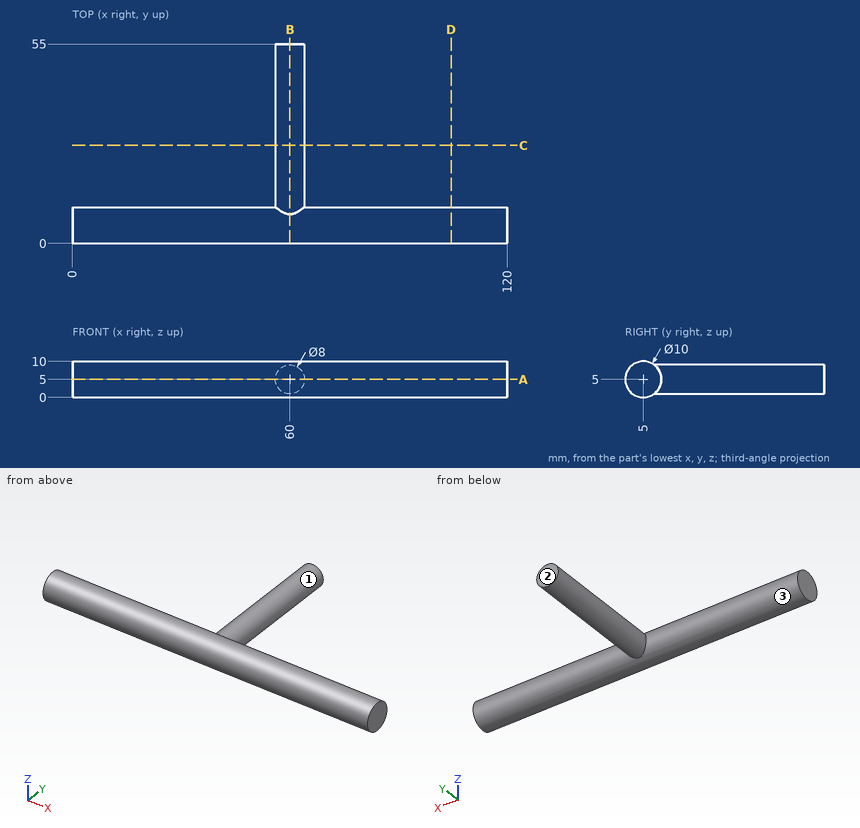
For this review, use the dimensioned drawing (mm, ordinates from the lowest corner) and the shaded views. A direction names the side the tool comes from. Give positions to 0.01 mm unless a question says otherwise; leave off trailing zeros. Write each loop counter-clockwise with the first axis right and the second up, starting at its lowest first coordinate (ties: lowest second). Pieces come first, ordered by that corner, then holes. Notation, with made-up numbers: M 82,-29 L 109,-29 A18 cw 109,-1 Z; hole C 43,54 d6. An arc over 180 degrees is marked long. Answer as a JSON object with one key per item and string values. Group by question number.
1) Clearance check with flat-ended pins moving along their axes: pin 1 Ø5 at (x, z) = (85, 5.5) entering from +Y; pin 2 Ø1.5 at (y, z) = (39, 7.5) entering from -X; pin 3 Ø5 at (x, z) = (106.5, 4.5) entering from -Y. State where each tip first meets the part, or that it passes through.
2) We need section D-D (x = 104.5). Give the boundary of the cut face in (y, z).
3) Tool access review of the marked faces 1, 2 and 3: name each direction out of +Z, -Z, +X, -X, +Y, -Y from which nothing blocks a thin tool from reaching the whole face with its end or side.
4) For line 1 along Y through (x, z) = (52.5, 5.5); line 2 along Y through (x, z) = (43, 2.25); line 3 along X through (y, z) = (50.5, 3.25), list the stretches that pass through material, from the lowest coordinate up.
5) We need section C-C (y = 27). Give the boundary of the cut face in (x, z), and give its area (3 significant figures).
6) We need section A-A (z = 5). Give the boundary of the cut face in (x, y).
7) We need section B-B (x = 60). Give the boundary of the cut face in (y, z), and give its area (3 significant figures).
Answer key:
{
 "1": {"pin 1": "stops at y = 10", "pin 2": "stops at x = 56.4", "pin 3": "stops at y = 0"},
 "2": {"outline": "C 5,5 d10"},
 "3": {"face 1": "+Y", "face 2": "+Z, -Z, +X, -X, +Y", "face 3": "none"},
 "4": {"line 1": "y = 0.03 to 9.97", "line 2": "y = 0.82 to 9.18", "line 3": "x = 56.4 to 63.6"},
 "5": {"outline": "C 60,5 d8", "area": "50.3 mm²"},
 "6": {"outline": "M 0,0 L 120,0 L 120,10 L 64,10 L 64,55 L 56,55 L 56,10 L 0,10 Z"},
 "7": {"outline": "M 8,1 L 55,1 L 55,9 L 8,9 A5 ccw long Z", "area": "443 mm²"}
}
